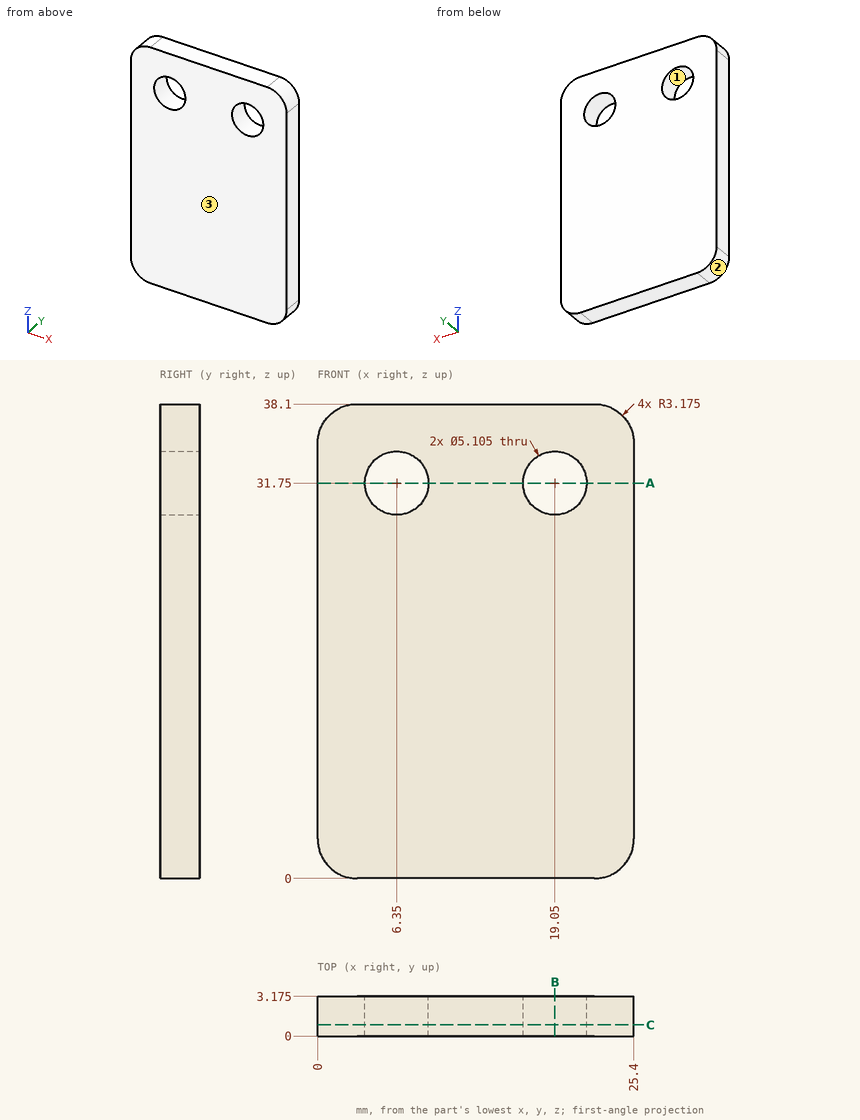
Design review of the part shown in the three views and the two pictorial views. Dimensions are in mm from the part's minimum x, y and z. Give positions to 0.01 mm unless a question says otherwise; leave off trailing zeros. Write each loop counter-clockwise with the first axis right and the second up, starting at its lowest first coordinate (ties: lowest second). Pieces come first, ordered by that corner, then holes.
Item 1: The part is to be moulded in two halves that separate along X. For the marked faces 1, 2 and 3, say which applies: +X half, -X half, draft (parallel to the pull), parting line (faces both ways), or undercut.
Item 2: Take a section at C-C (y = 0.9). Give the number of separate pieces and of enclosed holes in the cut face, and give its area (3 significant figures).
Item 3: Take a section at B-B (x = 19.05). Give the boundary of the cut face in (y, z) (1 decimal).
Item 4: Take a section at A-A (z = 31.75). Give the boundary of the cut face in (x, y) (1 decimal).
Item 5: Wall thickness on probe 1 along X at (y, z) = (1.9, 31.75); probe 2 along Z at (x, y) = (19.05, 1.4); probe 3 along X at (y, z) = (1.9, 30.5) (1 decimal): over which ranges is each line inside the solid? List them lowest first.
Established:
1. face 1: undercut
1. face 2: -X half
1. face 3: draft
2. separate pieces: 1
2. enclosed holes: 2
2. area: 918 mm2
3. outline: (0, 0) - (3.2, 0) - (3.2, 29.2) - (0, 29.2) - close; (0, 34.3) - (3.2, 34.3) - (3.2, 38.1) - (0, 38.1) - close
4. outline: (0, 0) - (3.8, 0) - (3.8, 3.2) - (0, 3.2) - close; (8.9, 0) - (16.5, 0) - (16.5, 3.2) - (8.9, 3.2) - close; (21.6, 0) - (25.4, 0) - (25.4, 3.2) - (21.6, 3.2) - close
5. probe 1: x = 0 to 3.8, 8.9 to 16.5, 21.6 to 25.4
5. probe 2: z = 0 to 29.2, 34.3 to 38.1
5. probe 3: x = 0 to 4.1, 8.6 to 16.8, 21.3 to 25.4
